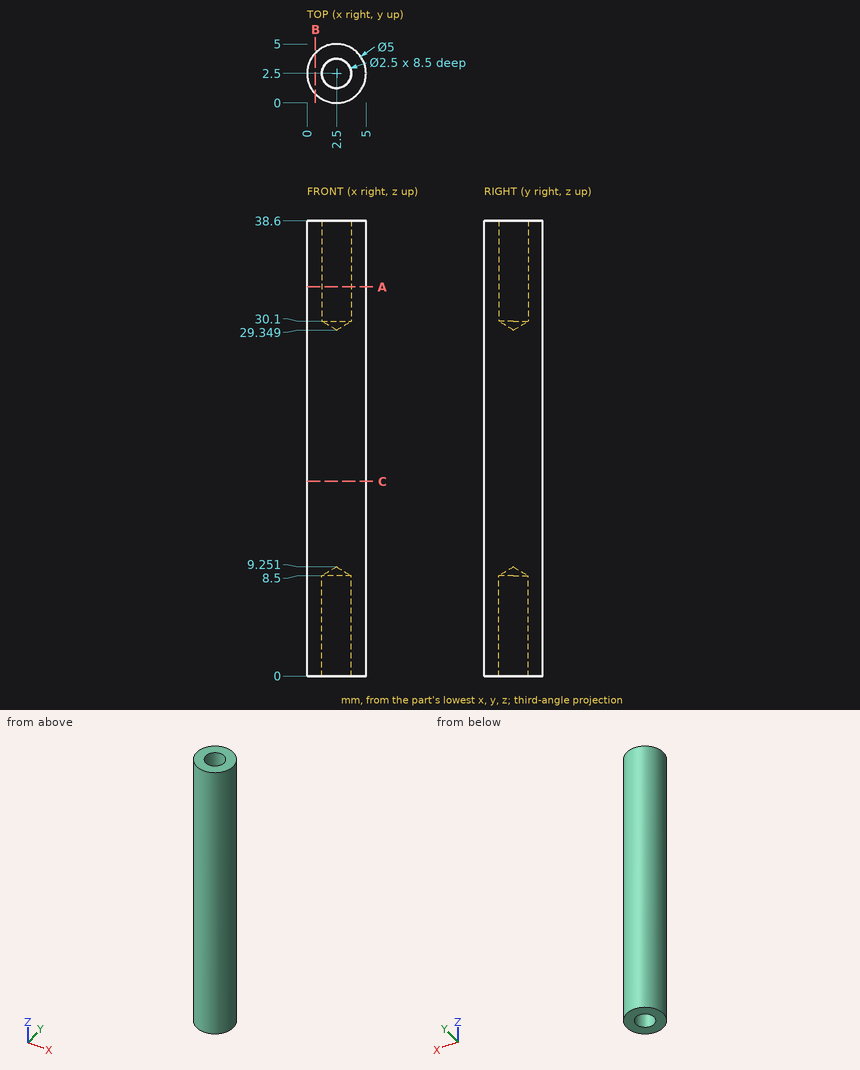
The drawing under review shows one solid part. Ordinate dimensions are in mm from its lowest x, y, z. Round coordinates to 2 decimals unless told otherwise and drop trailing zeros. Order: outer loops, then holes, each group sorted by start corner. A loop starts at its lowest first (then second) coordinate and runs counter-clockwise, first axis right, second up. Notation, with made-up numbers: (-33, 50) -> (-12, 50) arc R19 cw to (-12, 62) -> close; hole circle Ø8 at (23, 48). An arc over 180 degrees is marked (long way). Use a Markdown table: item, result.
Q1. We need section B-B on x = 0.7. Write out the cut boundary in (y, z) (3 decimals).
Values:
| item | result |
|---|---|
| outline | (0.765, 0) -> (4.235, 0) -> (4.235, 38.6) -> (0.765, 38.6) -> close |
Q2. We need section A-A on z = 33. Write out the cut boundary in (x, y), then the cut area to 3 significant figures.
Values:
| item | result |
|---|---|
| outline | circle Ø5 at (2.5, 2.5); hole circle Ø2.5 at (2.5, 2.5) |
| area | 14.7 mm^2 |
Q3. We need section C-C on z = 16.5. Write out the cut boundary in (x, y), then the cut area to 3 significant figures.
Values:
| item | result |
|---|---|
| outline | circle Ø5 at (2.5, 2.5) |
| area | 19.6 mm^2 |
Q4. For line 1 (Y direction, x = 2.5, z = 36.75); line 2 (Y direction, x = 2.35, z = 11), list the stretches that pass through material, from the lowest coordinate up.
Values:
| item | result |
|---|---|
| line 1 | y = 0 to 1.25, 3.75 to 5 |
| line 2 | y = 0 to 5 |
Q5. Clearance check with a flat-ended pin moving along its axis: P1, Ø1.5, axis at x = 2.5, y = 2.5, coming from the +Z side. State where the tip first meets the part, or that it passes through.
Values:
| item | result |
|---|---|
| P1 | stops at z = 29.8 |
